Could you check a few things on this drawing? It's one solid part, dimensions in mm from its lowest x, y, z. Round coordinates to 2 decimals unless told otherwise and drop trailing zeros. Loops run counter-clockwise (first coordinate to the right, second up) from the corner with the lowest first, then second, coordinate; pieces in that order, holes last. Notation, with made-up numbers: M -1,66 L 24,66 A24 ccw 24,105 Z; hole C 78,18 d1. An arc over 180 degrees is marked long. Return JSON: item names as keys, results as strings.
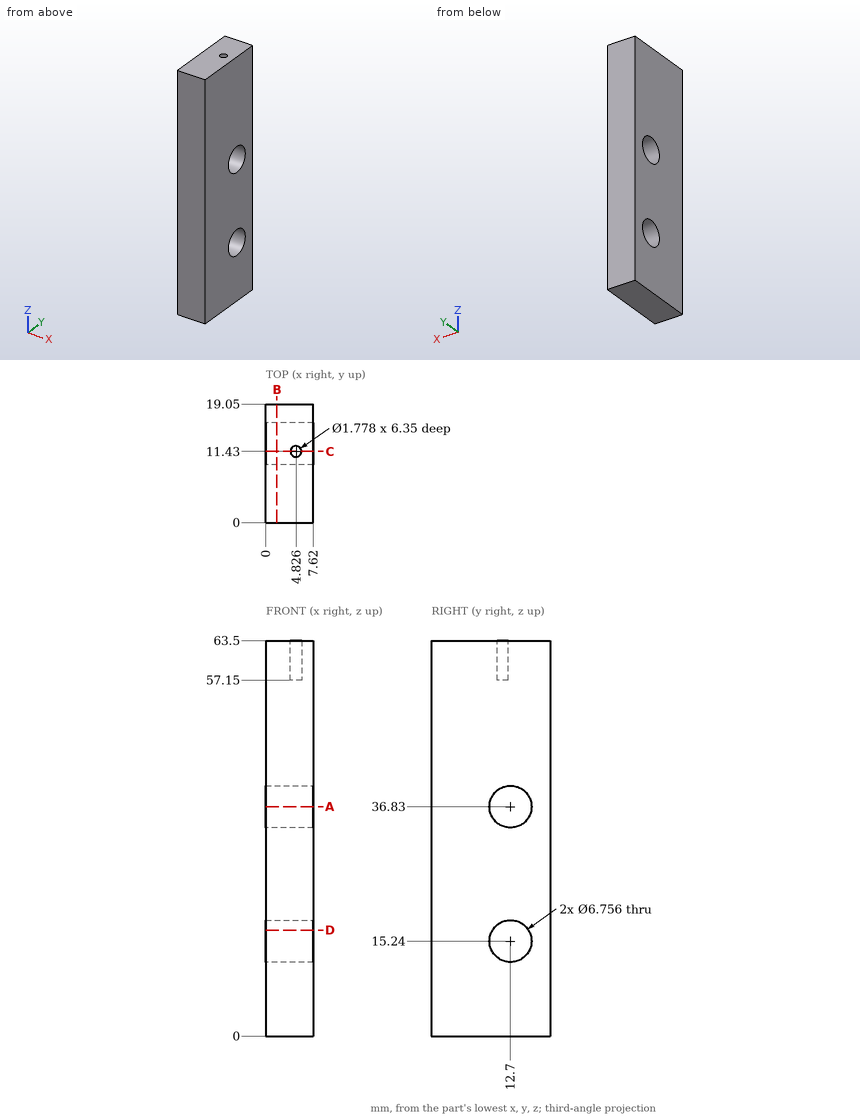
Q1. Suppose I cut it at A-A, the plane z = 36.83. Please give me the cut outline in (x, y).
Results:
{"outline": "M 0,0 L 7.62,0 L 7.62,9.32 L 0,9.32 Z; M 0,16.08 L 7.62,16.08 L 7.62,19.05 L 0,19.05 Z"}
Q2. If I drill on line 1 along Y through (x, z) = (5.25, 37); line 2 along Z through (x, y) = (5, 10.25) (1 decimal); line 3 along Z through (x, y) = (4.5, 14.25), over which ranges is the centre line in solid material (lowest first)?
Results:
{"line 1": "y = 0 to 9.33, 16.07 to 19.05", "line 2": "z = 0 to 12.9, 17.6 to 34.5, 39.2 to 63.5", "line 3": "z = 0 to 12.24, 18.24 to 33.83, 39.83 to 63.5"}
Q3. Suppose I cut it at B-B, the plane x = 1.75. Please give me the cut outline in (y, z).
Results:
{"outline": "M 0,0 L 19.05,0 L 19.05,63.5 L 0,63.5 Z; hole C 12.7,15.24 d6.76; hole C 12.7,36.83 d6.76"}
Q4. Suppose I cut it at D-D, the plane z = 17. Please give me the cut outline in (x, y), plus the area to 3 significant figures.
Results:
{"outline": "M 0,0 L 7.62,0 L 7.62,9.82 L 0,9.82 Z; M 0,15.58 L 7.62,15.58 L 7.62,19.05 L 0,19.05 Z", "area": "101 mm2"}
Q5. Suppose I cut it at C-C, the plane y = 11.43. State how many separate pieces and enclosed holes the cut face has, plus the area to 3 significant figures.
Results:
{"separate pieces": "3", "enclosed holes": "0", "area": "377 mm2"}
